from build123d import *

# Parameters (mm, degrees)
SKETCH_5_R      = 7.5
EXTRUDE_1_DEPTH = 10
SKETCH_5_3_R    = 45
SKETCH_5_3_R_2  = 12.5
SKETCH_5_3_R_3  = 7.5
SKETCH_5_3_R_4  = 22.5
SKETCH_5_3_R_5  = 4
SKETCH_5_3_R_6  = 6
EXTRUDE_2_DEPTH = 20
EXTRUDE_3_DEPTH = 15


with BuildPart() as part:
    # Sketch 5 → Extrude 1 (new body)
    with BuildSketch(Plane.XY):
        with BuildLine():
            ThreePointArc((187, 0), (176.748737342, 24.748737342), (152, 35))
            Line((152, 35), (32.249030993, 35))
            ThreePointArc((32.249030993, 35), (28.694937727, 35.538393609), (25.45976131, 37.105263158))
            ThreePointArc((25.45976131, 37.105263158), (39.816386444, 20.967960571), (45, 0))
            ThreePointArc((45, 0), (43.758881795, -10.495725989), (40.103988265, -20.41249924))
            ThreePointArc((40.103988265, -20.41249924), (45.898229653, -14.901907218), (53.868271349, -14.255151415))
            Line((53.868271349, -14.255151415), (128.412955316, -33.981898358))
            Line((128.412955316, -33.981898358), (168.162642233, -44.500851195))
            ThreePointArc((168.162642233, -44.500851195), (181.149853373, -41.886134075), (187, -30))
            Line((187, -30), (187, 0))
        make_face()
        with Locations((172, -30)):
            Circle(SKETCH_5_R, mode=Mode.SUBTRACT)
        with BuildLine():
            Line((90.497574655, 20), (152, 20))
            ThreePointArc((152, 20), (171.832919165, -2.579790186), (146.883522978, -19.33446826))
            Line((146.883522978, -19.33446826), (87.427688442, -3.600680956))
            ThreePointArc((87.427688442, -3.600680956), (78.597823156, 9.547874112), (90.497574655, 20))
        make_face(mode=Mode.SUBTRACT)
    extrude(amount=EXTRUDE_1_DEPTH)

    # Sketch 5_3 → Extrude 2 (add)
    # profile 1 of 2: a face of its own
    with BuildSketch(Plane.XY):
        with Locations(Location((0, 0, 0), (0, 0, 55.544049539))):
            Circle(SKETCH_5_3_R)
        Circle(SKETCH_5_3_R_2, mode=Mode.SUBTRACT)
        with Locations((-25.980762114, 15)):
            Circle(SKETCH_5_3_R_3, mode=Mode.SUBTRACT)
        with Locations((-25.980762114, -15)):
            Circle(SKETCH_5_3_R_3, mode=Mode.SUBTRACT)
        with Locations((0, -30)):
            Circle(SKETCH_5_3_R_3, mode=Mode.SUBTRACT)
        with Locations((25.980762114, -15)):
            Circle(SKETCH_5_3_R_3, mode=Mode.SUBTRACT)
        with Locations((25.980762114, 15)):
            Circle(SKETCH_5_3_R_3, mode=Mode.SUBTRACT)
        with Locations((0, 30)):
            Circle(SKETCH_5_3_R_3, mode=Mode.SUBTRACT)
    # profile 2 of 2: a face of its own
    with BuildSketch(Plane.XY):
        with Locations((94, -60)):
            Circle(SKETCH_5_3_R_4)
        with Locations((103.899494937, -69.899494937)):
            Circle(SKETCH_5_3_R_5, mode=Mode.SUBTRACT)
        with Locations((103.899494937, -50.100505063)):
            Circle(SKETCH_5_3_R_5, mode=Mode.SUBTRACT)
        with Locations((84.100505063, -50.100505063)):
            Circle(SKETCH_5_3_R_5, mode=Mode.SUBTRACT)
        with Locations((84.100505063, -69.899494937)):
            Circle(SKETCH_5_3_R_5, mode=Mode.SUBTRACT)
        with Locations((94, -60)):
            Circle(SKETCH_5_3_R_6, mode=Mode.SUBTRACT)
    extrude(amount=EXTRUDE_2_DEPTH)


with BuildPart() as extrude_2_piece_1:
    # of the separate pieces the step leaves, piece 1, a body of its own (extrude_2_pieces)
    add(part.part.solids().sort_by_distance((168.162642233, -44.500851195, 0))[0])



with BuildPart() as extrude_2_piece_2:
    # of the separate pieces the step leaves, piece 2, a body of its own (extrude_2_pieces)
    add(part.part.solids().sort_by_distance((116.5, -60, 0))[0])


with BuildPart() as extrude_2_piece_1_1:
    add(extrude_2_piece_1.part)

    add(extrude_2_piece_2.part)  # Extrude 3 merges Extrude 2 piece 2
    # Sketch 5_4 → Extrude 3 (add)
    with BuildSketch(Plane.XY):
        with BuildLine():
            ThreePointArc((40.103988265, -20.41249924), (2.027406196, -44.954305957), (-38.103740681, -23.9396104))
            ThreePointArc((-38.103740681, -23.9396104), (21.140554647, -74.43017402), (98.610149033, -82.02263667))
            ThreePointArc((98.610149033, -82.02263667), (73.905745166, -49.877207764), (114.441132023, -50.597334335))
            ThreePointArc((114.441132023, -50.597334335), (116.158656581, -37.859460343), (128.412955316, -33.981898358))
            Line((128.412955316, -33.981898358), (53.868271349, -14.255151415))
            ThreePointArc((53.868271349, -14.255151415), (45.898229653, -14.901907218), (40.103988265, -20.41249924))
        make_face()
    extrude(amount=EXTRUDE_3_DEPTH)


solid = extrude_2_piece_1_1.part
Model file for the job. Use its own axes, mm. A direction names the side the tool comes from. Round coordinates to 2 decimals unless told otherwise and drop trailing zeros. Order: outer loops, then holes, each group sorted by start corner. A loop starts at its lowest first (then second) coordinate and runs counter-clockwise, first axis right, second up.
(1) Drill centre lines: line 1 (Y direction, x = 0, z = 15.5); line 2 (Y direction, x = 0.5, z = 9.25); line 3 (Y direction, x = -31.5, z = 2). Where is each one in solid material? Low to high.
(2) Band-saw the part on B-B (y = 30). List the corners of the cut face in (x, z).
(3) 3-axis set-ups, long thin cutter, end or side, ignore diameter. For faces 1 (the face through (114.784, -68.618, 12.082)), 2 (the face through (78.57, 9.31, 4.93)), 3 (the face through (13, 2, 20)): which of +Z, -Z, +X, -X, +Y, -Y reach the whole face in a straight line?
(4) Band-saw the part on D-D (y = 15). List the corners of the cut face in (x, z).
(5) Band-saw the part on C-C (x = 22.5). List the corners of the cut face in (y, z), then the cut area to 3 significant figures.
(6) Pull direction Y, two halves, no side cores. Call faces 4 (the face through (177.019, 24.475, 4.93)), 5 (the face through (181, -42, 5)), 6 (the face through (44, -49, 15)), 7 (the face through (80.104, -49.925, 9.86)): released by +Y, released by -Y, zero draft, split by the parting line, or undercut.
(7) Band-saw the part on A-A (z = 17.75). Give the number of separate pieces and of enclosed holes in the cut face, then the cut area to 3 significant figures.
(8) Pin check, flat tips, straight feed: pin 1 (11 mm diameter, centred on x = 124.5, z = 5.5, fed in from -Y); pin 2 (9 mm diameter, centred on x = 84.1, y = -50.1, fed in from +Z); pin 3 (21.5 mm diameter, centred on x = 48, y = -33.5, fed in from +Z); pin 4 (12 mm diameter, centred on x = 53, z = 10.5, fed in from -Y). Stop position of each tip, or through.
Verdict:
1. line 1: y = -45 to -37.5, -22.5 to -12.5, 12.5 to 22.5, 37.5 to 45
1. line 2: y = -63.37 to -37.48, -22.52 to -12.49, 12.49 to 22.52, 37.48 to 45
1. line 3: y = -33.48 to -20.08, -9.92 to 9.92, 20.08 to 32.14
2. outline: (-33.54, 0) - (-7.5, 0) - (-7.5, 20) - (-33.54, 20) - close; (7.5, 0) - (170.03, 0) - (170.03, 10) - (33.54, 10) - (33.54, 20) - (7.5, 20) - close
3. face 1: +Z
3. face 2: +Z, -Z
3. face 3: +Z, +X, -X, +Y, -Y
4. outline: (-42.43, 0) - (-33.48, 0) - (-33.48, 20) - (-42.43, 20) - close; (-18.48, 0) - (18.48, 0) - (18.48, 20) - (-18.48, 20) - close; (33.48, 0) - (80.75, 0) - (80.75, 10) - (42.43, 10) - (42.43, 20) - (33.48, 20) - close; (165.23, 0) - (183.62, 0) - (183.62, 10) - (165.23, 10) - close
5. outline: (-75, 0) - (-21.64, 0) - (-21.64, 20) - (-38.97, 20) - (-38.97, 15) - (-75, 15) - close; (-8.36, 0) - (8.36, 0) - (8.36, 20) - (-8.36, 20) - close; (21.64, 0) - (38.97, 0) - (38.97, 20) - (21.64, 20) - close
5. area: 1,570 mm2
6. face 4: released by +Y
6. face 5: released by -Y
6. face 6: zero draft
6. face 7: undercut
7. separate pieces: 2
7. enclosed holes: 12
7. area: 6,090 mm2
8. pin 1: stops at y = -35.4
8. pin 2: stops at z = 20
8. pin 3: stops at z = 15
8. pin 4: stops at y = -84.13
